The listing builds one solid part. Answer for the finished solid, in the listing's coordinates (mm). A direction names the side the tool comes from. Round coordinates to 2 decimals unless told otherwise and drop trailing zeros. Loops run counter-clockwise (first coordinate to the right, second up) from the corner with the lowest first, then second, coordinate; pieces in that order, holes last. Notation, with made-up numbers: (89, 57) - (132, 57) arc R14 cw to (132, 77) - close; hole circle Ø11 at (28.25, 77.25). An arc over 180 degrees is marked (long way). One line per question, with ' | ' between items. Start each with the question number.
from build123d import *

# Parameters (mm, degrees)
F0_R     = 4
F0_R_2   = 3.4
F1_DEPTH = 10


with BuildPart() as f1:
    # F0 (on Right) → F1 (new body)
    with BuildSketch(Plane.YZ):
        with BuildLine():
            Line((47.677108, -50.710301), (83.328195, -45.710301))
            ThreePointArc((83.328195, -45.710301), (89.485461, -42.368894), (91.939306, -35.807221))
            Line((91.939306, -35.807221), (91.939306, 24.192779))
            ThreePointArc((91.939306, 24.192779), (88.490403, 31.748117), (80.522681, 34.091929))
            Line((80.522681, 34.091929), (67.093321, 32.17011))
            ThreePointArc((67.093321, 32.17011), (65.074623, 32.087401), (63.080502, 32.412149))
            ThreePointArc((63.080502, 32.412149), (61.944816, 32.791702), (60.86264, 33.30428))
            Line((60.86264, 33.30428), (4.3249, 64.356929))
            ThreePointArc((4.3249, 64.356929), (3.435792, 64.830914), (2.503502, 65.213024))
            ThreePointArc((2.503502, 65.213024), (-9.142416, 61.321845), (-8.237688, 49.076432))
            Line((-8.237688, 49.076432), (15.086959, 23.262908))
            ThreePointArc((15.086959, 23.262908), (15.818861, 20.750279), (14.29987, 18.619163))
            Line((14.29987, 18.619163), (-18.293867, 0.804326))
            ThreePointArc((-18.293867, 0.804326), (-23.497782, -7.960254), (-18.311843, -16.735482))
            Line((-18.311843, -16.735482), (41.474164, -49.572201))
            ThreePointArc((41.474164, -49.572201), (44.48357, -50.643035), (47.677108, -50.710301))
        make_face()
        with Locations((-13.497787, -7.970503)):
            Circle(F0_R, mode=Mode.SUBTRACT)
        with BuildLine():
            ThreePointArc((31.849396, 5.418782), (34.818502, 5.366689), (36.28822, 2.786334))
            Line((36.28822, 2.786334), (36.28822, -18.835382))
            ThreePointArc((36.28822, -18.835382), (34.815857, -21.417304), (31.844003, -21.464876))
            Line((31.844003, -21.464876), (12.112738, -10.627725))
            ThreePointArc((12.112738, -10.627725), (10.556957, -7.995156), (12.118131, -5.365782))
            Line((12.118131, -5.365782), (31.849396, 5.418782))
        make_face(mode=Mode.SUBTRACT)
        with Locations((46.28822, -40.807221)):
            Circle(F0_R_2, mode=Mode.SUBTRACT)
        with Locations((58.171915, -39.140554)):
            Circle(F0_R_2, mode=Mode.SUBTRACT)
        with Locations((70.055611, -37.473888)):
            Circle(F0_R_2, mode=Mode.SUBTRACT)
        with Locations((46.28822, -30.807221)):
            Circle(F0_R_2, mode=Mode.SUBTRACT)
        with Locations((58.171915, -29.140554)):
            Circle(F0_R_2, mode=Mode.SUBTRACT)
        with Locations((70.055611, -27.473888)):
            Circle(F0_R_2, mode=Mode.SUBTRACT)
        with Locations((81.939306, -35.807221)):
            Circle(F0_R_2, mode=Mode.SUBTRACT)
        with BuildLine():
            ThreePointArc((78.588797, -26.385221), (78.580112, -26.332397), (78.572259, -26.279443))
            ThreePointArc((78.572259, -26.279443), (81.702621, -22.415469), (85.339306, -25.807221))
            ThreePointArc((85.339306, -25.807221), (82.229364, -29.194826), (78.588797, -26.385221))
        make_face(mode=Mode.SUBTRACT)
        with Locations((46.28822, -20.807221)):
            Circle(F0_R_2, mode=Mode.SUBTRACT)
        with Locations((58.171915, -19.140554)):
            Circle(F0_R_2, mode=Mode.SUBTRACT)
        Polygon((58.171915, -9.503709), (57.880681, -9.181399), (58.171915, -9.140554), align=None, mode=Mode.SUBTRACT)
        with Locations((70.055611, -17.473888)):
            Circle(F0_R_2, mode=Mode.SUBTRACT)
        with Locations((46.28822, -0.807221)):
            Circle(F0_R_2, mode=Mode.SUBTRACT)
        with Locations((58.171915, 0.859446)):
            Circle(F0_R_2, mode=Mode.SUBTRACT)
        with BuildLine():
            ThreePointArc((70.725603, -0.807221), (70.392261, -0.85718), (70.055611, -0.873888))
            ThreePointArc((70.055611, -0.873888), (69.718961, -0.85718), (69.385619, -0.807221))
            ThreePointArc((69.385619, -0.807221), (67.90131, 5.156509), (73.455611, 2.526112))
            ThreePointArc((73.455611, 2.526112), (72.686007, 0.371811), (70.725603, -0.807221))
        make_face(mode=Mode.SUBTRACT)
        with Locations((81.939306, -15.807221)):
            Circle(F0_R_2, mode=Mode.SUBTRACT)
        with Locations((81.939306, 4.192779)):
            Circle(F0_R_2, mode=Mode.SUBTRACT)
        with Locations((-0.817978, 55.780752)):
            Circle(F0_R, mode=Mode.SUBTRACT)
        with Locations((46.28822, 9.192779)):
            Circle(F0_R_2, mode=Mode.SUBTRACT)
        with Locations((58.171915, 10.859446)):
            Circle(F0_R_2, mode=Mode.SUBTRACT)
        with Locations((46.28822, 19.192779)):
            Circle(F0_R_2, mode=Mode.SUBTRACT)
        with Locations((58.171915, 20.859446)):
            Circle(F0_R_2, mode=Mode.SUBTRACT)
        with Locations((70.055611, 12.526112)):
            Circle(F0_R_2, mode=Mode.SUBTRACT)
        with Locations((70.055611, 22.526112)):
            Circle(F0_R_2, mode=Mode.SUBTRACT)
        with Locations((81.939306, 14.192779)):
            Circle(F0_R_2, mode=Mode.SUBTRACT)
        with Locations((81.939306, 24.192779)):
            Circle(F0_R_2, mode=Mode.SUBTRACT)
    extrude(amount=F1_DEPTH)


solid = f1.part
(1) Each of these flat-tipped pins is pushed along its axis until it touches: P1, Ø4, axis at y = 70.06, z = 2.53, coming from the +X side; P2, Ø4, axis at x = 5, z = -31.5, coming from the -Y side; P3, Ø4, axis at x = 7, z = 53, coming from the +Y side; P4, Ø3, axis at x = 5, y = 41.5, coming from the -Z side. Where does it stop, or does it pass through?
(2) Find section C-C on x = 5.25. Count the separate pieces of the cut face and the enclosed holes in it, plus the area to 3 significant figures.
(3) Find section A-A on y = -3.5. Write down the section's boundary in (x, z).
(4) Determine the mould class of faces 1 (the cylindrical face through (4.93, 85.182, -14.786)), 2 (the flat face through (5, 91.939, -6)), 3 (the flat face through (4.93, 22.116, -16.122)), 4 (the cylindrical face through (4.93, -23.497, -7.811)) for opening direction Y: pulls with the +Y half, pulls with the -Y half, needs draft (parallel to the pull), parting line crosses it, or undercut.
(5) Consider L1, parallel to Z at x = 1.5, y = 13.5; L2, parallel to Y at x = 2.25, z = -28.5; L3, parallel to Y at x = 5.5, z = -25.5. Determine where each line is inside the solid, lowest interval first.
(6) Find section B-B on y = 22. Write down the section's boundary in (x, z).
(7) A tool of negligible diameter and unlimited length cuts with its end or side. For faces 5 (the cylindrical face through (4.93, 10.557, -8.04)), 6 (the flat face through (4.93, 11.163, -32.924)), 7 (the flat face through (4.93, 3.26, 36.35)), from which of +Z, -Z, +X, -X, +Y, -Y can it reach the whole face along a straight path? Write none if from no direction.
(8) Find section D-D on z = 30.5. Write down the section's boundary in (x, y), plus the area to 3 significant figures.
Answer below:
1) P1: through | P2: y = 4.93 | P3: y = 28.64 | P4: z = -50.25
2) separate pieces: 1 | enclosed holes: 28 | area: 7,140 mm2
3) outline: (0, -24.87) - (10, -24.87) - (10, 8.89) - (0, 8.89) - close; (0, 43.83) - (10, 43.83) - (10, 52.81) - (0, 52.81) - close; (0, 58.75) - (10, 58.75) - (10, 65.41) - (0, 65.41) - close
4) face 1: undercut | face 2: pulls with the +Y half | face 3: undercut | face 4: pulls with the -Y half
5) L1: -34.21 to -11.39, -4.61 to 18.18, 25.02 to 59.32 | L2: 3.11 to 43.79, 48.79 to 54.83, 61.51 to 66.81, 73.3 to 79.86, 84.02 to 91.94 | L3: -2.35 to 67.29, 72.82 to 78.55, 85.33 to 91.94
6) outline: (0, -38.88) - (10, -38.88) - (10, -16.06) - (0, -16.06) - close; (0, 0.04) - (10, 0.04) - (10, 54.65) - (0, 54.65) - close
7) face 5: +X, -X | face 6: -Z, +X, -X, -Y | face 7: +X, -X, -Y
8) outline: (0, 8.55) - (10, 8.55) - (10, 89.7) - (0, 89.7) - close | area: 812 mm2
